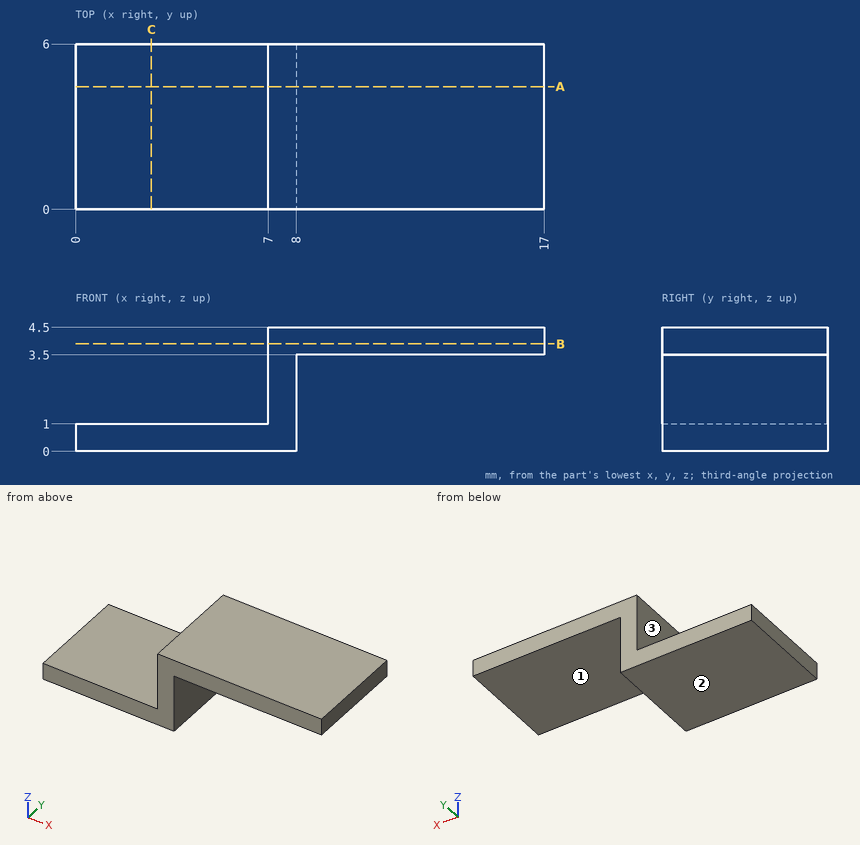
Geometry: see drawing. Coordinates: mm, zero at the bounding-box minimum. A direction names the side the tool comes from. Coordinates: 2 decimals unless noted, no trailing zeros. Write each loop counter-clockwise with the first axis right and the second up, starting at its lowest first coordinate (ties: lowest second). Pieces come first, ordered by that corner, then holes. Notation, with made-up numbers: M 61,-30.5 L 102,-30.5 A12 ccw 102,-7.5 Z; hole C -36.5,-10 d10. An arc over 180 degrees is marked long. Use CSV: the item, a comma, the result in double quotes. Start each with the question number.
1. First-contact query: P1, Ø2, axis at y = 3.5, z = 1, coming from the +X side; P2, Ø3, axis at x = 4.5, y = 2.5, coming from the -Z side; P3, Ø1, axis at y = 3, z = 2.5, coming from the -X side. Flat tips, straight axial feed; report the tip coordinate or a pass-through.
2. Cut plane C-C on x = 2.75. Return the cut outline in (y, z).
3. Cut plane A-A on y = 4.45. Return the cut outline in (x, z).
4. Cut plane B-B on z = 3.9. Return the cut outline in (x, y).
5. Reachability of the marked faces 1, 2 and 3 from +Z, -Z, +X, -X, +Y, -Y: full face, straight path, thin tool, end or side. Return the list, or none.
6. Ray query, probe 1 along Z at (x, y) = (15, 0.35); probe 2 along X at (y, z) = (3.9, 1.5); probe 3 along Z at (x, y) = (1.25, 1.7). Return the intervals inside material, ascending.
Entries:
1,P1,"x = 8"
1,P2,"z = 0"
1,P3,"x = 7"
2,outline,"M 0,0 L 6,0 L 6,1 L 0,1 Z"
3,outline,"M 0,0 L 8,0 L 8,3.5 L 17,3.5 L 17,4.5 L 7,4.5 L 7,1 L 0,1 Z"
4,outline,"M 7,0 L 17,0 L 17,6 L 7,6 Z"
5,face 1,"-Z, +X, +Y, -Y"
5,face 2,"-Z, +X, -X, +Y, -Y"
5,face 3,"+Z, -X, +Y, -Y"
6,probe 1,"3.5 to 4.5"
6,probe 2,"7 to 8"
6,probe 3,"0 to 1"
